CAD build for the part. Positions are in the model's coordinates, mm. Face numbers are marked on the shaded views. A direction names the side the tool comes from. Round coordinates to 2 decimals unless told otherwise and drop trailing zeros. Loops run counter-clockwise (first coordinate to the right, second up) from the corner with the lowest first, then second, coordinate; pieces in that order, holes last. Notation, with made-up numbers: M 77.25,9 L 130.25,9 A25 cw 130.25,43 Z; hole C -9.75,82 d4. An arc over 180 degrees is marked long. Use a Markdown table: item, result. Add a question column.
(1) Band-saw the part on B-B, the plane y = 32. Write the cut outline in (x, z).
(2) Band-saw the part on A-A, the plane z = 24.5. Write the cut outline in (x, y).
(3) Wall check: L1, parallel to Z at x = 9.5, y = 29.5; L2, parallel to X at y = 11.5, z = 41; L3, parallel to Z at x = 3.5, y = 12. Give the ranges that are in metal, low to high.
(4) Band-saw the part on D-D, the plane z = 32.5. Write the cut outline in (x, y).
(5) Two-plate mould, pull along Z, no slides. Class the marked faces 1, 2 and 3: released by +Z, released by -Z, zero draft, split by the parting line, or undercut.
(6) Which spindle directions (+Z, -Z, +X, -X, +Y, -Y) get a long thin tool onto all of the face, cutting with end or side? Do the marked faces 4, 5 and 6. Say none if no direction does.
(7) Band-saw the part on C-C, the plane x = 7. Write the cut outline in (y, z), and give its area (3 significant figures).
(8) Flat gauge pins, fed straight in: P1, Ø1.5, axis at x = 7.5, y = 4, coming from the +Z side; P2, Ø1.5, axis at x = 12.5, z = 42.5, coming from the +Y side; P3, Ø3, axis at x = 9, y = -9.5, coming from the -Z side. Where does each tip first touch, or does it go through?
from build123d import *

# Parameters (mm, degrees)
EXTRUDE_START       = -18
SKETCH_1_W          = 13.648314944
SKETCH_1_H          = 27.972083639
EXTRUDE_1_DEPTH     = 33
SKETCH_3_W          = 18
SKETCH_3_H          = 34
EXTRUDE_2_DEPTH     = 30
SKETCH_4_W          = 20.982707523
SKETCH_4_H          = 19.792714352
CUT_EXTRUDE_1_DEPTH = 22
FILLET_1_R          = 4
SKETCH_5_R          = 2.5
CUT_EXTRUDE_2_DEPTH = 60.029924153
CHAMFER_1_SIZE      = 4


with BuildPart() as part:
    # Эскиз1 → Вытянуть1 (new body)
    with BuildSketch(Plane(origin=(0, 0, 0), x_dir=(1, 0, 0), z_dir=(0, 1, 0)).offset(EXTRUDE_START)):
        with Locations((8.422168222, -36.610171765)):
            Rectangle(SKETCH_1_W, SKETCH_1_H)
    extrude(amount=EXTRUDE_1_DEPTH)

    # Эскиз3 → Вытянуть2 (add)
    with BuildSketch(Plane(origin=(0, 15, 0), x_dir=(1, 0, 0), z_dir=(0, 1, 0))):
        with Locations((8.422168222, -36.610171766)):
            Rectangle(SKETCH_3_W, SKETCH_3_H)
    extrude(amount=EXTRUDE_2_DEPTH)

    # Эскиз4 → Вырез-Вытянуть1 (cut)
    with BuildSketch(Plane(origin=(0, 45, 0), x_dir=(1, 0, 0), z_dir=(0, 1, 0))):
        with Locations((9.143949352, -37.062876014)):
            Rectangle(SKETCH_4_W, SKETCH_4_H)
    extrude(amount=-CUT_EXTRUDE_1_DEPTH, mode=Mode.SUBTRACT)

    # Скругление1
    fillet_1_edges = [part.edges().sort_by_distance(p)[0] for p in [
        (8.422168222, 23, 27.166518838),
        (8.422168222, 23, 46.95923319),
    ]]
    fillet(fillet_1_edges, radius=FILLET_1_R)

    # Эскиз5 → Вырез-Вытянуть2 (cut, through all)
    with BuildSketch(Plane.XY.offset(53.610171766)):
        with Locations((8.422168222, 37)):
            Circle(SKETCH_5_R)
    extrude(amount=-CUT_EXTRUDE_2_DEPTH, mode=Mode.SUBTRACT)

    # Фаска1
    chamfer_1_edges = [part.edges().sort_by_distance(p)[0] for p in [
        (-0.577831778, 45, 23.388345302),
        (17.422168222, 45, 50.284702478),
        (-0.577831778, 45, 50.284702478),
        (17.422168222, 45, 23.388345302),
    ]]
    chamfer(chamfer_1_edges, length=CHAMFER_1_SIZE)


solid = part.part
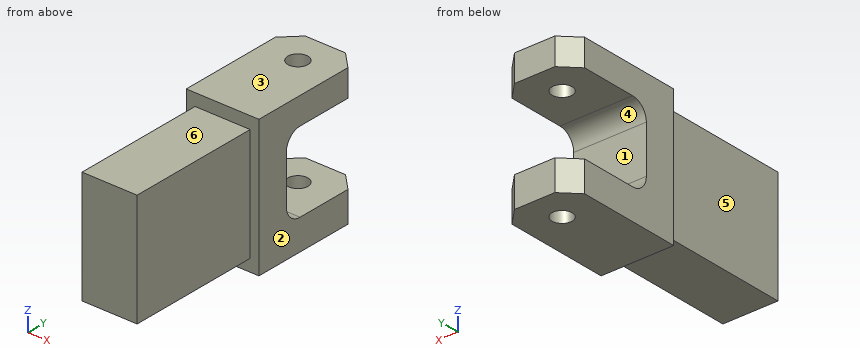
Return value:
| question | item | result |
|---|---|---|
| 1 | outline | M -0.58,19.61 L 17.42,19.61 L 17.42,27.17 L -0.58,27.17 Z; M -0.58,46.96 L 17.42,46.96 L 17.42,53.61 L -0.58,53.61 Z |
| 2 | outline | M -0.58,15 L 1.6,15 L 1.6,-18 L 15.25,-18 L 15.25,15 L 17.42,15 L 17.42,41 L 13.42,45 L 3.42,45 L -0.58,41 Z; hole C 8.42,37 d5 |
| 3 | L1 | 19.61 to 27.17, 46.96 to 53.61 |
| 3 | L2 | 1.6 to 15.25 |
| 3 | L3 | 22.62 to 50.6 |
| 4 | outline | M -0.58,15 L 1.6,15 L 1.6,-18 L 15.25,-18 L 15.25,15 L 17.42,15 L 17.42,23 L -0.58,23 Z |
| 5 | face 1 | undercut |
| 5 | face 2 | zero draft |
| 5 | face 3 | released by +Z |
| 6 | face 4 | +X, -X, +Y |
| 6 | face 5 | +Z, -Z, -X, -Y |
| 6 | face 6 | +Z, +X, -X, -Y |
| 7 | outline | M -18,22.62 L 15,22.62 L 15,19.61 L 34.94,19.61 L 34.94,27.17 L 27,27.17 A4 cw 23,31.17 L 23,42.96 A4 cw 27,46.96 L 34.94,46.96 L 34.94,53.61 L 15,53.61 L 15,50.6 L -18,50.6 Z; M 39.06,19.61 L 45,19.61 L 45,27.17 L 39.06,27.17 Z; M 39.06,46.96 L 45,46.96 L 45,53.61 L 39.06,53.61 Z |
| 7 | area | 1,460 mm^2 |
| 8 | P1 | z = 50.6 |
| 8 | P2 | y = 23.01 |
| 8 | P3 | z = 22.62 |
